Input: part model. Units: mm. Frame: model coordinates. A direction names the side the tool comes from. Coordinates: 2 decimals unless noted, no trailing zeros. Order: outer loops, then holes, each group sorted by start corner. A loop starts at its lowest first (then second) coordinate and runs counter-clockwise, first axis right, second up.
from build123d import *

# Parameters (mm, degrees)
F0_W     = 114.3
F0_H     = 31.75
F1_DEPTH = 11.1125
F2_W     = 38.1
F2_H     = 31.75
F3_DEPTH = 6.35
F5_DEPTH = 6.35


# Not quite as in the source:
# - a feature of the source that left no trace in its solid (it failed there, or was rolled back) is left out
# - a pattern or mirror of a feature is missing from the dataset's text; its kind, count and spacing are read off the source's solid


with BuildPart() as f1:
    # F0 (on Top) → F1 (new body, symmetric)
    with BuildSketch(Plane.XY):
        Rectangle(F0_W, F0_H)
    extrude(amount=F1_DEPTH, both=True)

    # F2 (on face) → F3 (cut)
    with BuildSketch(Plane.XY.offset(11.1125)):
        with Locations((-38.1, 0)):
            Rectangle(F2_W, F2_H)
    f3 = extrude(amount=-F3_DEPTH, mode=Mode.SUBTRACT)

    # F3_copies: F3 across plane
    add(f3.mirror(Plane(origin=(0, 0, 0), x_dir=(-1, 0, 0), z_dir=(0, 0, -1))), mode=Mode.SUBTRACT)

    # F4 (on face) → F5 (cut)
    with BuildSketch(Plane.XY.offset(11.1125)):
        Polygon((57.15, -15.875), (57.15, 15.875), (12.7, 15.875), (19.05, -15.875), align=None)
    f5 = extrude(amount=-F5_DEPTH, mode=Mode.SUBTRACT)

    # F5_copies: F5 across plane
    add(f5.mirror(Plane(origin=(0, 0, 0), x_dir=(-1, 0, 0), z_dir=(0, 0, -1))), mode=Mode.SUBTRACT)


solid = f1.part
Item 1: Cut plane C-C on z = -9.5. Return loops of the section in (x, y) (3 decimals).
Response values:
outline: (-19.05, -15.875) - (19.05, -15.875) - (12.7, 15.875) - (-19.05, 15.875) - close
Item 2: Ray query, probe 1 along Z at (x, y) = (49, -5); probe 2 along X at (y, z) = (14.5, 6.5) (3 decimals); probe 3 along X at (y, z) = (6, 7.75) (3 decimals). Return the intervals inside material, ascending.
Response values:
probe 1: z = -4.76 to 4.76
probe 2: x = -19.05 to 12.975
probe 3: x = -19.05 to 14.675
Item 3: Cut plane B-B on x = 15. Return loops of the section in (y, z) (1 decimal), then the cut area to 3 significant figures.
Response values:
outline: (-15.9, -11.1) - (4.4, -11.1) - (4.4, -4.8) - (15.9, -4.8) - (15.9, 4.8) - (4.4, 4.8) - (4.4, 11.1) - (-15.9, 11.1) - close
area: 560 mm2
Item 4: Pin query (flat end, axial travel): pin 1 Ø4 at (y, z) = (-1, -8) entering from +X (3 decimals); pin 2 Ø9.5 at (x, y) = (37, 6.5) entering from +Z; pin 3 Ø5 at (y, z) = (-5.5, -9) entering from -X. Return the tip coordinate at first contact, or that it passes through.
Response values:
pin 1: stops at x = 16.475
pin 2: stops at z = 4.76
pin 3: stops at x = -19.05
Item 5: Access query for faces 1 (the face through (-38, 0, 4.763)), 2 (the face through (-38, 0, -4.763)), 3 (the face through (15.83, 0.22, -7.98)). Directions: +Z, -Z, +X, -X, +Y, -Y. A direction counts if a zero-diameter tool reaches every point of the face in a straight line with its end or side. Return the directions, or none.
Response values:
face 1: +Z, -X, +Y, -Y
face 2: -Z, -X, +Y, -Y
face 3: -Z, +X, +Y
